Verification items for the finished model (mm, model axes). A direction names the side the tool comes from. Give positions to 0.01 mm unless a question says otherwise; leave off trailing zeros. Write each loop counter-clockwise with the first axis right and the second up, starting at its lowest first coordinate (ties: lowest second). Pieces come first, ordered by that corner, then holes. Notation, with made-up numbers: (-35.75, 32) -> (-26.75, 32) arc R28 cw to (-26.75, 71) -> close; hole circle Ø8 at (-14, -36). An arc over 180 degrees is marked (long way). Use one line per item in the form item = value. Start each with the question number.
(1) Depth check by flat-ended pin: pin 1 Ø1.5 at (y, z) = (42, 9.5) entering from -X; pin 2 Ø0.6 at (x, y) = (0, -1.5) entering from -Z; pin 3 Ø4 at (x, y) = (2, 62) entering from -Z; pin 4 Ø3 at (x, z) = (-8, 34) entering from +Y. Enter the tip coordinate at first touch or a pass-through.
(2) Section check D-D, the plane y = 75.8. State how many separate pieces and enclosed holes the cut face has, plus the area to 3 significant figures.
(3) Section check C-C, the plane y = 125. Record the cut outline in (x, z).
(4) Release check for a two-part mould opening along X. For faces 5 (the face through (-5, 90, -24)), 6 (the face through (10, 87.5, 30)), 7 (the face through (25, 69, 22)) record: pulls with the +X half, pulls with the -X half, needs draft (parallel to the pull), parting line crosses it, or undercut.
(5) Set-up check for faces 1 (the face through (-11, 96, -32.5)), 2 (the face through (-15, 91, -30)), 3 (the face through (1.3, 3, 28.7)), 4 (the face through (-28.7, 3, -1.3)): record each of +Z, -Z, +X, -X, +Y, -Y from which the full face is reachable in a straight line by a thin tool's end or side.
(6) Section check B-B, the plane x = 13. Record the cut outline in (y, z).
(7) Section check A-A, the plane z = 7. Record the cut outline in (x, y).
(8) Scan lines: L1, parallel to Z at x = 22.9, y = 75.8; L2, parallel to Z at x = 21, y = 78. Record each from-to range of solid material in increasing order.
from build123d import *

# Parameters (mm, degrees)
SKETCH1_W                = 50
SKETCH1_H                = 50
SKETCH1_W_2              = 42
SKETCH1_H_2              = 42
BOSS_EXTRUDE1_DEPTH      = 140.8
CUT_EXTRUDE1_DEPTH       = 152.491385894
SKETCH5_W                = 10
SKETCH5_H                = 10
BOSS_EXTRUDE3_DEPTH      = 15
SKETCH8_W                = 10
SKETCH8_H                = 10
CUT_EXTRUDE4_DEPTH       = 107.56570743
SKETCH9_W                = 30
SKETCH9_H                = 5
CUT_EXTRUDE5_DEPTH       = 5
SKETCH10_R               = 1.25
CUT_EXTRUDE6_DEPTH       = 10
FILLET5_R                = 1
FILLET6_R                = 1
CUT_EXTRUDE3_REACH       = 155.459
SKETCH7_W                = 42
SKETCH7_H                = 42
SKETCH11_W               = 3
SKETCH11_H               = 86.5
BOSS_EXTRUDE4_DEPTH      = 8
CUT_EXTRUDE11_REACH      = 154.508
SKETCH16_R               = 1.5
FILLET3_R                = 3
FILLET4_R                = 0.5
BOSS_EXTRUDE6_DEPTH      = 4
BOSS_EXTRUDE6_DEPTH_BACK = 3
SKETCH18_W               = 6
SKETCH18_H               = 8
SKETCH18_R               = 1.5
SKETCH18_W_2             = 8
SKETCH18_H_2             = 6
FILLET7_R                = 2


with BuildPart() as part:
    # Sketch1 → Boss-Extrude1 (new body)
    with BuildSketch(Plane(origin=(0, 0, 0), x_dir=(1, 0, 0), z_dir=(0, 1, 0))):
        Rectangle(SKETCH1_W, SKETCH1_H)
        Rectangle(SKETCH1_W_2, SKETCH1_H_2, mode=Mode.SUBTRACT)
    extrude(amount=BOSS_EXTRUDE1_DEPTH)

    # Sketch3 → Cut-Extrude1 (cut, through all)
    with BuildSketch(Plane(origin=(0, 0, -25), x_dir=(-1, 0, 0), z_dir=(0, 0, -1))):
        with BuildLine():
            Line((-5, 140.8), (5, 140.8))
            Line((5, 140.8), (5, 38))
            ThreePointArc((5, 38), (0, 33), (-5, 38))
            Line((-5, 38), (-5, 140.8))
        make_face()
    extrude(amount=-CUT_EXTRUDE1_DEPTH, mode=Mode.SUBTRACT)

    # Sketch5 → Boss-Extrude3 (add, symmetric)
    with BuildSketch(Plane(origin=(0, 0, 25), x_dir=(0, 0, 1), z_dir=(-1, 0, 0))):
        with Locations((5, 92.5)):
            Rectangle(SKETCH5_W, SKETCH5_H)
    boss_extrude3 = extrude(amount=BOSS_EXTRUDE3_DEPTH, both=True)

    # Sketch8 → Cut-Extrude4 (cut, through all)
    with BuildSketch(Plane(origin=(0, 97.5, 0), x_dir=(1, 0, 0), z_dir=(0, 1, 0))):
        with Locations((0, -30)):
            Rectangle(SKETCH8_W, SKETCH8_H)
    cut_extrude4 = extrude(amount=-CUT_EXTRUDE4_DEPTH, mode=Mode.SUBTRACT)

    # Sketch9 → Cut-Extrude5 (cut)
    with BuildSketch(Plane(origin=(0, 97.5, 0), x_dir=(1, 0, 0), z_dir=(0, 1, 0))):
        with Locations((0, -30)):
            Rectangle(SKETCH9_W, SKETCH9_H)
    cut_extrude5 = extrude(amount=-CUT_EXTRUDE5_DEPTH, mode=Mode.SUBTRACT)

    # Sketch10 → Cut-Extrude6 (cut)
    with BuildSketch(Plane.XY.offset(35)):
        with Locations((-10, 95)):
            Circle(SKETCH10_R)
        with Locations((10, 95)):
            Circle(SKETCH10_R)
    cut_extrude6 = extrude(amount=-CUT_EXTRUDE6_DEPTH, mode=Mode.SUBTRACT)

    # Fillet5
    fillet5_edges = [part.edges().sort_by_distance(p)[0] for p in [
        (5, 97.5, 26.25),
        (5, 119.15, 25),
        (-5, 62.75, 25),
        (0, 33, 25),
        (5, 62.75, 25),
        (-5, 119.15, 25),
        (-10, 97.5, 25),
        (-10, 87.5, 25),
        (15, 92.5, 25),
        (10, 87.5, 25),
        (10, 97.5, 25),
        (-15, 92.5, 25),
        (5, 87.5, 30),
        (-5, 87.5, 30),
        (-5, 97.5, 26.25),
    ]]
    fillet(fillet5_edges, radius=FILLET5_R)

    # Mirror7: Boss-Extrude3, Cut-Extrude4, Cut-Extrude5, Cut-Extrude6 across plane
    add(boss_extrude3.mirror(Plane.XY))
    add(cut_extrude4.mirror(Plane.XY), mode=Mode.SUBTRACT)
    add(cut_extrude5.mirror(Plane.XY), mode=Mode.SUBTRACT)
    add(cut_extrude6.mirror(Plane.XY), mode=Mode.SUBTRACT)

    # Fillet6
    fillet6_edges = [part.edges().sort_by_distance(p)[0] for p in [
        (5, 62.75, -25),
        (-5, 119.15, -25),
        (-10, 87.5, -25),
        (-10, 97.5, -25),
        (10, 97.5, -25),
        (-15, 92.5, -25),
        (10, 87.5, -25),
        (15, 92.5, -25),
        (-5, 97.5, -26.25),
        (-5, 87.5, -30),
        (5, 87.5, -30),
        (5, 97.5, -26.25),
        (5, 119.15, -25),
        (0, 33, -25),
        (-5, 62.75, -25),
    ]]
    fillet(fillet6_edges, radius=FILLET6_R)

    # Sketch7 → Cut-Extrude3 (cut, up to next)
    with BuildSketch(Plane(origin=(25, 0, 0), x_dir=(0, 0, -1), z_dir=(1, 0, 0)), mode=Mode.PRIVATE) as cut_extrude3_sk1:
        with Locations((0, 73)):
            Rectangle(SKETCH7_W, SKETCH7_H)
    cut_extrude3_tool1 = extrude(cut_extrude3_sk1.sketch, amount=-CUT_EXTRUDE3_REACH, mode=Mode.PRIVATE) & part.part
    add(cut_extrude3_tool1.solids().sort_by_distance((25, 73, 0))[0], mode=Mode.SUBTRACT)

    # Sketch11 → Boss-Extrude4 (add)
    with BuildSketch(Plane.XY.offset(25)):
        with Locations((23.5, 97.55)):
            Rectangle(SKETCH11_W, SKETCH11_H)
    boss_extrude4 = extrude(amount=BOSS_EXTRUDE4_DEPTH)

    # Sketch16 → Cut-Extrude11 (cut, up to next)
    with BuildSketch(Plane.ZY.offset(-22), mode=Mode.PRIVATE) as cut_extrude11_sk1:
        with Locations(Location((29, 120.8, 0), (0, 0, 270))):
            Circle(SKETCH16_R)
    cut_extrude11_tool1 = extrude(cut_extrude11_sk1.sketch, amount=-CUT_EXTRUDE11_REACH, mode=Mode.PRIVATE) & part.part
    # Sketch16 → Cut-Extrude11 (cut, up to next)
    with BuildSketch(Plane.ZY.offset(-22), mode=Mode.PRIVATE) as cut_extrude11_sk2:
        with Locations(Location((29, 75.8, 0), (0, 0, 270))):
            Circle(SKETCH16_R)
    cut_extrude11_tool2 = extrude(cut_extrude11_sk2.sketch, amount=-CUT_EXTRUDE11_REACH, mode=Mode.PRIVATE) & part.part
    cut_extrude11_1 = cut_extrude11_tool1.solids().sort_by_distance((22, 120.8, 29))[0]
    add(cut_extrude11_1, mode=Mode.SUBTRACT)
    cut_extrude11_2 = cut_extrude11_tool2.solids().sort_by_distance((22, 75.8, 29))[0]
    add(cut_extrude11_2, mode=Mode.SUBTRACT)
    cut_extrude11 = cut_extrude11_1 + cut_extrude11_2  # Cut-Extrude11 as one shape, for the pattern or mirror that repeats it

    # Mirror8: Boss-Extrude4, Cut-Extrude11 across plane
    add(boss_extrude4.mirror(Plane.XY))
    add(cut_extrude11.mirror(Plane.XY), mode=Mode.SUBTRACT)

    # Fillet3
    fillet3_edges = [part.edges().sort_by_distance(p)[0] for p in [
        (-25, 70.4, -25),
        (-25, 70.4, 25),
    ]]
    fillet(fillet3_edges, radius=FILLET3_R)

    # Fillet4
    fillet4_edges = [part.edges().sort_by_distance(p)[0] for p in [
        (22, 97.55, 33),
        (22, 97.55, -33),
    ]]
    fillet(fillet4_edges, radius=FILLET4_R)

    # Sketch18 → Boss-Extrude6 (add, two sides: drawn at the far end of the back side and taken through both)
    # profile 1 of 3: a face of its own
    with BuildSketch(Plane.XZ.offset(-BOSS_EXTRUDE6_DEPTH_BACK)):
        with Locations((0, 29)):
            Rectangle(SKETCH18_W, SKETCH18_H)
        with Locations(Location((0, 30, 0), (0, 0, 270))):
            Circle(SKETCH18_R, mode=Mode.SUBTRACT)
    # profile 2 of 3: a face of its own
    with BuildSketch(Plane.XZ.offset(-BOSS_EXTRUDE6_DEPTH_BACK)):
        with Locations((-29, 0)):
            Rectangle(SKETCH18_W_2, SKETCH18_H_2)
        with Locations(Location((-30, 0, 0), (0, 0, 270))):
            Circle(SKETCH18_R, mode=Mode.SUBTRACT)
    # profile 3 of 3: a face of its own
    with BuildSketch(Plane.XZ.offset(-BOSS_EXTRUDE6_DEPTH_BACK)):
        with Locations((0, -29)):
            Rectangle(SKETCH18_W, SKETCH18_H)
        with Locations(Location((0, -30, 0), (0, 0, 270))):
            Circle(SKETCH18_R, mode=Mode.SUBTRACT)
    extrude(amount=BOSS_EXTRUDE6_DEPTH + BOSS_EXTRUDE6_DEPTH_BACK)

    # Fillet7
    fillet7_edges = [part.edges().sort_by_distance(p)[0] for p in [
        (-25, 3, 0),
        (-25, 1.5, 3),
        (-25, 1.5, -3),
        (-33, -0.5, -3),
        (-33, -0.5, 3),
        (0, 3, 25),
        (3, 1.5, 25),
        (-3, 1.5, 25),
        (-3, -0.5, 33),
        (3, -0.5, 33),
        (0, 3, -25),
        (-3, 1.5, -25),
        (3, 1.5, -25),
        (3, -0.5, -33),
        (-3, -0.5, -33),
    ]]
    fillet(fillet7_edges, radius=FILLET7_R)


solid = part.part
Completed:
q1.pin_1 = -25
q1.pin_2 = -33
q1.pin_3 = through
q1.pin_4 = 97.5
q2.separate_pieces = 5
q2.enclosed_holes = 0
q2.area = 513 mm²
q3.outline = (-25, -22) arc R3 ccw to (-22, -25) -> (-6, -25) arc R1 ccw to (-5, -24) -> (-5, -21) -> (-21, -21) -> (-21, 21) -> (-5, 21) -> (-5, 24) arc R1 ccw to (-6, 25) -> (-22, 25) arc R3 ccw to (-25, 22) -> close; (5, -24) arc R1 ccw to (6, -25) -> (22, -25) -> (22, -32.5) arc R0.5 ccw to (22.5, -33) -> (25, -33) -> (25, 33) -> (22.5, 33) arc R0.5 ccw to (22, 32.5) -> (22, 25) -> (6, 25) arc R1 ccw to (5, 24) -> (5, 21) -> (21, 21) -> (21, -21) -> (5, -21) -> close
q4.face_5 = undercut
q4.face_6 = needs draft
q4.face_7 = pulls with the +X half
q5.face_1 = -X, +Y
q5.face_2 = -Z, -X, +Y, -Y
q5.face_3 = +Z, +X, -X, +Y
q5.face_4 = +Z, -Z, -X, +Y
q6.outline = (0, -25) -> (86.5, -25) arc R1 cw to (87.5, -26) -> (87.5, -35) -> (97.5, -35) -> (97.5, -32.5) -> (92.5, -32.5) -> (92.5, -27.5) -> (97.5, -27.5) -> (97.5, -26) arc R1 cw to (98.5, -25) -> (140.8, -25) -> (140.8, -21) -> (0, -21) -> close; (0, 21) -> (140.8, 21) -> (140.8, 25) -> (98.5, 25) arc R1 cw to (97.5, 26) -> (97.5, 27.5) -> (92.5, 27.5) -> (92.5, 32.5) -> (97.5, 32.5) -> (97.5, 35) -> (87.5, 35) -> (87.5, 26) arc R1 cw to (86.5, 25) -> (0, 25) -> close
q7.outline = (-25, 0) -> (-21, 0) -> (-21, 140.8) -> (-25, 140.8) -> close; (21, 0) -> (25, 0) -> (25, 52) -> (21, 52) -> close; (21, 94) -> (25, 94) -> (25, 140.8) -> (21, 140.8) -> close
q8.L1 = -33 to -30.5, -27.5 to -21, 21 to 27.5, 30.5 to 33
q8.L2 = -25 to -21, 21 to 25
